```python
from build123d import *

# Parameters (mm, degrees)
F0_R     = 32.5
F0_R_2   = 20
F1_DEPTH = 37.5
F2_R     = 25
F2_R_2   = 20
F3_DEPTH = 17
F4_R     = 25
F4_R_2   = 20
F5_DEPTH = 17


with BuildPart() as f1:
    # F0 (on Right) → F1 (new body, symmetric)
    with BuildSketch(Plane.YZ):
        Circle(F0_R)
        Circle(F0_R_2, mode=Mode.SUBTRACT)
    extrude(amount=F1_DEPTH, both=True)

    # F2 (on face) → F3 (cut)
    with BuildSketch(Plane.YZ.offset(37.5)):
        Circle(F2_R)
        Circle(F2_R_2, mode=Mode.SUBTRACT)
    extrude(amount=-F3_DEPTH, mode=Mode.SUBTRACT)

    # F4 (on face) → F5 (cut)
    with BuildSketch(Plane(origin=(-37.5, 0, 0), x_dir=(0, -1, 0), z_dir=(-1, 0, 0))):
        Circle(F4_R)
        Circle(F4_R_2, mode=Mode.SUBTRACT)
    extrude(amount=-F5_DEPTH, mode=Mode.SUBTRACT)


solid = f1.part
```
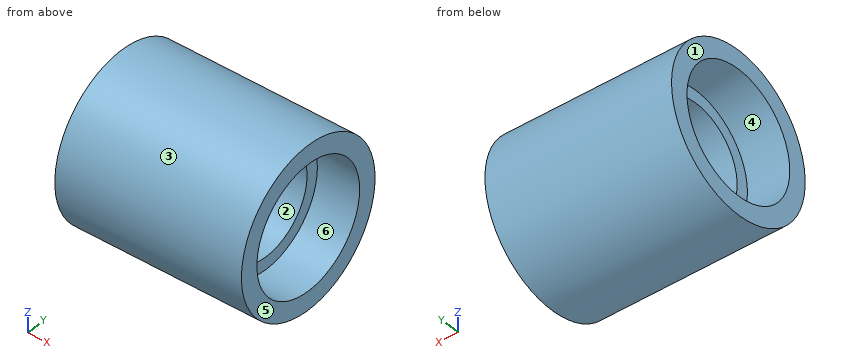
Input: part model. Units: mm. Frame: model coordinates. Face numbers are marked on the shaded views. A direction names the side the tool comes from. Coordinates: 2 decimals unless noted, no trailing zeros. Loops run counter-clockwise (first coordinate to the right, second up) from the corner with the lowest first, then second, coordinate; pieces in that order, holes last. Notation, with made-up numbers: M -23,1.5 L -6,1.5 A17 ccw -6,5.5 Z; hole C -28,44 d9. An arc over 180 degrees is marked long. Use a Markdown table: item, result. Add a question column.
1) Line query: L1, parallel to Z at x = 5, y = 0; L2, parallel to Z at x = -25.75, y = 0; L3, parallel to Y at x = -13.5, z = -3.5. Output: solid intervals per line, ascending. Write a range as from..to.
2) Section A-A, the plane z = 0. Return the cut outline in (x, y).
3) Section B-B, the plane x = 33. Return the cut outline in (y, z).
4) Section D-D, the plane z = 21. Return the cut outline in (x, y), plus the area to 3 significant figures.
5) Draft query along Y for the marked faces 1, 2 and 3. Return one class per face: +Y half, -Y half, draft (parallel to the pull), parting line (faces both ways), or undercut.
6) Section C-C, the plane y = 6. Return the cut outline in (x, z), plus the area to 3 significant figures.
7) Pin query (flat end, axial travel): P1, Ø5, axis at x = 24, z = 7.5, coming from the +Y side; P2, Ø12, axis at x = -20, y = 13, coming from the +Z side; P3, Ø1, axis at x = 26, y = 13, coming from the +Z side; P4, Ø1, axis at y = -13.5, z = 13, coming from the +X side. Return the tip coordinate at first contact, or that it passes through.
8) Set-up query: the marked faces 4, 5 and 6. Return all of +Z, -Z, +X, -X, +Y, -Y with unobstructed straight access to the full face (end or side cutting, diameter ignored); none if empty.
Answer below:
| question | item | result |
|---|---|---|
| 1 | L1 | -32.5..-20, 20..32.5 |
| 1 | L2 | -32.5..-25, 25..32.5 |
| 1 | L3 | -32.31..-19.69, 19.69..32.31 |
| 2 | outline | M -37.5,-32.5 L 37.5,-32.5 L 37.5,-25 L 20.5,-25 L 20.5,-20 L -20.5,-20 L -20.5,-25 L -37.5,-25 Z; M -37.5,25 L -20.5,25 L -20.5,20 L 20.5,20 L 20.5,25 L 37.5,25 L 37.5,32.5 L -37.5,32.5 Z |
| 3 | outline | C 0,0 d65; hole C 0,0 d50 |
| 4 | outline | M -37.5,-24.8 L 37.5,-24.8 L 37.5,-13.56 L 20.5,-13.56 L 20.5,13.56 L 37.5,13.56 L 37.5,24.8 L -37.5,24.8 L -37.5,13.56 L -20.5,13.56 L -20.5,-13.56 L -37.5,-13.56 Z |
| 4 | area | 2,800 mm2 |
| 5 | face 1 | draft |
| 5 | face 2 | undercut |
| 5 | face 3 | parting line |
| 6 | outline | M -37.5,-31.94 L 37.5,-31.94 L 37.5,-24.27 L 20.5,-24.27 L 20.5,-19.08 L -20.5,-19.08 L -20.5,-24.27 L -37.5,-24.27 Z; M -37.5,24.27 L -20.5,24.27 L -20.5,19.08 L 20.5,19.08 L 20.5,24.27 L 37.5,24.27 L 37.5,31.94 L -37.5,31.94 Z |
| 6 | area | 1,580 mm2 |
| 7 | P1 | y = 32.11 |
| 7 | P2 | z = 31.74 |
| 7 | P3 | z = 30 |
| 7 | P4 | through |
| 8 | face 4 | -X |
| 8 | face 5 | +Z, -Z, +X, +Y, -Y |
| 8 | face 6 | +X |
